Can you work these out from the model? Positions are in its coordinate system, mm. Face numbers are marked on the shaded views. A direction names the side the tool comes from. Coordinates: 2 decimals unless noted, no trailing zeros. Order: outer loops, then holes, each group sorted by start corner. A loop starts at its lowest first (then second) coordinate and runs counter-clockwise, first axis right, second up.
Autodesk Inventor part; units mm, degrees
ref_plane "YZ Plane" through (0, 0, 0) normal (1, 0, 0) x (0, 1, 0)
ref_plane "XZ Plane" through (0, 0, 0) normal (0, 1, 0) x (-1, 0, 0)
ref_plane "XY Plane" through (0, 0, 0) normal (0, 0, 1) x (1, 0, 0)
sketch "Sketch1" plane through (0, 0, 0) normal (0, 0, 1) x (1, 0, 0)
  arc A0 (0, 7.5) -> (6.8483, -3.0578) centre (0, 0) ccw
  line L0 (0, 7.5) -> (23.5, 7.5)
  line L1 (23.5, 7.5) -> (23.5, 4.5)
  line L2 (23.5, 4.5) -> (18.5, 4.5)
  arc A1 (18.5, 4.5) -> (6.8483, -3.0578) centre (18.5, -8.2604) ccw
  dimension "d0" = 15
  dimension "d3" = 3
  dimension "d5" = 23.5
  dimension "d12" = 5
extrude "Extrusion1" add sketch "Sketch1" along normal blind 28
shell "Shell1" thickness 0.18 removed faces 1 at (23.5, 5.5, 18.6667)
sketch "Sketch2" plane through (0, 0, 28) normal (0, 0, 1) x (1, 0, 0)
  circle A0 centre (0, 0) radius 4
  dimension "d9" = 8
extrude "Extrusion2" cut sketch "Sketch2" against normal blind 31
properties part number "blower"
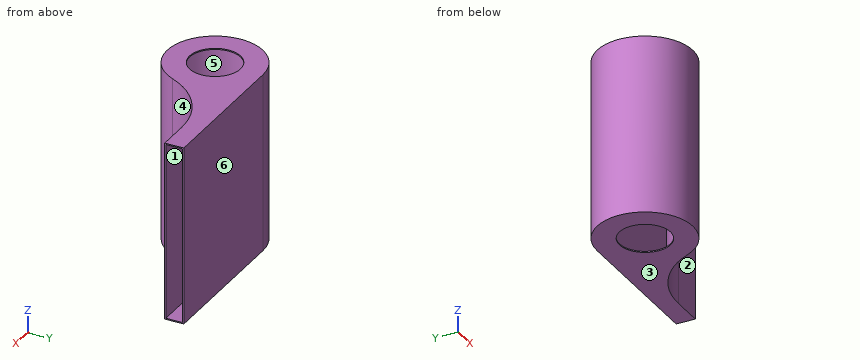
1. Thinking about a two-plate mould opening in Y: for the marked faces 4, 5 and 6, which applies, pulls with the +Y half, pulls with the -Y half, needs draft (parallel to the pull), parting line crosses it, or undercut?
Completed:
face 4: pulls with the -Y half
face 5: undercut
face 6: pulls with the +Y half
2. I'm going to push flat-ended pins straight in: pin 1 (2.5 mm diameter, centred on x = 21.5, z = 15, fed in from -Y); pin 2 (7 mm diameter, centred on x = 0, y = 0, fed in from +Z); pin 3 (12 mm diameter, centred on x = 15.5, z = 12, fed in from -Y); pin 4 (5 mm diameter, centred on y = 1, z = 16.5, fed in from +X). Where does each tip first touch, or does it pass through?
Completed:
pin 1: stops at y = 4.5
pin 2: passes through
pin 3: stops at y = 0.79
pin 4: stops at x = 13.55
3. Imagine slicing it at B-B on z = 4. Please give me the cut outline in (x, y), then the cut area to 3 significant figures.
Completed:
outline: (0, 7.32) - (23.5, 7.32) - (23.5, 7.5) - (0, 7.5) arc R7.5 ccw (long way) to (6.85, -3.06) arc R12.76 cw to (18.5, 4.5) - (23.5, 4.5) - (23.5, 4.68) - (18.5, 4.68) arc R12.94 ccw to (6.68, -2.98) arc R7.32 cw (long way) to start
area: 13.5 mm2
4. Imagine slicing it at D-D on x = 0.5. Please give me the cut outline in (y, z).
Completed:
outline: (-7.48, 0) - (-3.97, 0) - (-3.97, 0.18) - (-7.3, 0.18) - (-7.3, 27.82) - (-3.97, 27.82) - (-3.97, 28) - (-7.48, 28) - close; (3.97, 0) - (7.5, 0) - (7.5, 28) - (3.97, 28) - (3.97, 27.82) - (7.32, 27.82) - (7.32, 0.18) - (3.97, 0.18) - close
5. Imagine slicing it at C-C on x = 17.5. Please give me the cut outline in (y, z), then the cut area to 3 significant figures.
Completed:
outline: (4.46, 0) - (7.5, 0) - (7.5, 28) - (4.46, 28) - close; hole (4.64, 0.18) - (7.32, 0.18) - (7.32, 27.82) - (4.64, 27.82) - close
area: 11.1 mm2
6. Please list where these lines run through material, in increasing order: probe 1 along Z at (x, y) = (17.5, 6.25); probe 2 along Y at (x, z) = (20, 26.5); probe 3 along Y at (x, z) = (0, 27.95).
Completed:
probe 1: z = 0 to 0.18, 27.82 to 28
probe 2: y = 4.5 to 4.68, 7.32 to 7.5
probe 3: y = -7.5 to -4, 4 to 7.5
7. Imagine slicing it at A-A on y = 0. Please give me the cut outline in (x, z).
Completed:
outline: (-7.5, 0) - (-4, 0) - (-4, 0.18) - (-7.32, 0.18) - (-7.32, 27.82) - (-4, 27.82) - (-4, 28) - (-7.5, 28) - close; (4, 0) - (8.77, 0) - (8.77, 28) - (4, 28) - (4, 27.82) - (8.54, 27.82) - (8.54, 0.18) - (4, 0.18) - close
8. On a 3-axis mill with a long thin cutter (end or side, diameter ignored), from which of +Z, -Z, +X, -X, +Y, -Y can I reach the whole of each face in a straight line? I mean the marked faces 1, 2 and 3. Say none if no direction works.
Completed:
face 1: +X
face 2: +Z, -Z, +X, -Y
face 3: -Z, +X, -X, +Y, -Y
